from build123d import *

# Parameters (mm, degrees)
SKETCH1_R           = 6.25
BOSS_EXTRUDE1_DEPTH = 30
CUT_EXTRUDE3_DEPTH  = 15
SKETCH9_W           = 12.5
SKETCH9_H           = 25
BOSS_EXTRUDE2_DEPTH = 3
SKETCH11_W          = 10.933781676
SKETCH11_H          = 25
SKETCH11_W_2        = 11.938681189
CUT_EXTRUDE4_DEPTH  = 34
SKETCH12_R          = 6.25
BOSS_EXTRUDE3_DEPTH = 5
CHAMFER1_SIZE       = 1


with BuildPart() as part:
    # Sketch1 → Boss-Extrude1 (new body)
    with BuildSketch(Plane.XY):
        Circle(SKETCH1_R)
    extrude(amount=BOSS_EXTRUDE1_DEPTH)

    # Sketch8 → Cut-Extrude3 (cut)
    with BuildSketch(Plane(origin=(0, 0, 0), x_dir=(-1, 0, 0), z_dir=(0, 0, -1))):
        with BuildLine():
            Line((-1.616322988, 2.1), (1.616322988, 2.1))
            ThreePointArc((1.616322988, 2.1), (0, -2.65), (-1.616322988, 2.1))
        make_face()
    extrude(amount=-CUT_EXTRUDE3_DEPTH, mode=Mode.SUBTRACT)

    # Sketch9 → Boss-Extrude2 (add)
    with BuildSketch(Plane.XY.offset(30)):
        Rectangle(SKETCH9_W, SKETCH9_H)
    extrude(amount=BOSS_EXTRUDE2_DEPTH)

    # Sketch10 → Revolve1 (revolve)
    with BuildSketch(Plane(origin=(0, 0, 0), x_dir=(0, 0, -1), z_dir=(1, 0, 0))):
        Polygon((-30, 12.5), (-30, 0), (-17.5, 0), align=None)
    revolve(axis=Axis((0, 0, 63.541170981), (0, 0, 1)))

    # Sketch11 → Cut-Extrude4 (cut, through all)
    with BuildSketch(Plane.XY.offset(33)):
        with Locations((-11.716890838, 0)):
            Rectangle(SKETCH11_W, SKETCH11_H)
        with Locations((12.219340595, 0)):
            Rectangle(SKETCH11_W_2, SKETCH11_H)
    extrude(amount=-CUT_EXTRUDE4_DEPTH, mode=Mode.SUBTRACT)

    # Sketch12 → Boss-Extrude3 (add)
    with BuildSketch(Plane.XY.offset(33)):
        Circle(SKETCH12_R)
    extrude(amount=BOSS_EXTRUDE3_DEPTH)

    # Chamfer1
    chamfer1_edges = [part.edges().sort_by_distance(p)[0] for p in [
        (-6.25, 0, 38),
    ]]
    chamfer(chamfer1_edges, length=CHAMFER1_SIZE)


solid = part.part
Could you check a few things on this model? Use its own coordinates, in mm. A direction names the side the tool comes from. Coordinates: 2 decimals unless noted, no trailing zeros. Order: outer loops, then holes, each group sorted by start corner. A loop starts at its lowest first (then second) coordinate and runs counter-clockwise, first axis right, second up.
Q1. Thinking about a two-plate mould opening in Y: for faces 1 (the flat face through (5, 12, 30)), 2 (the flat face through (0, 2.1, 7)), 3 (the conical face through (0.2, 8.7, 26.2)), 4 (the cylindrical face through (-0.09, -2.65, 7.4)), which applies, released by +Y, released by -Y, zero draft, split by the parting line, or undercut?
Q2. Suppose I cut it at B-B on z = 26. Please give me the cut outline in (x, y), and give its area (3 significant figures).
Q3. Please list where these lines run through material, in increasing order: L1, parallel to Y at x = 0, z = 9.5; L2, parallel to X at y = 0, z = 4; L3, parallel to Y at x = -1, z = 11.
Q4. Will these pins go through, and if not, where does the flat tip stop? pin 1 (4 mm diameter, centred on x = -3.5, y = 9.5, fed in from -Z); pin 2 (2 mm diameter, centred on x = 2, z = 6, fed in from +Y); pin 3 (1.5 mm diameter, centred on y = -3.5, z = 11.5, fed in from +X).
Q5. Suppose I cut it at A-A on z = 34.5. Please give me the cut outline in (x, y), and give its area (3 significant figures).
Q6. Which directions (+Z, -Z, +X, -X, +Y, -Y) give clear straight access to the entire face, cutting with the end or side of a thin tool? Please do faces 5 (the cylindrical face through (5.96, 1.88, 11.71)), 6 (the flat face through (0, -9, 33)), 7 (the flat face through (-5, 12, 30)).
Answer:
1. face 1: zero draft
1. face 2: undercut
1. face 3: released by +Y
1. face 4: undercut
2. outline: (-6.25, -5.76) arc R8.5 ccw to (6.25, -5.76) - (6.25, 5.76) arc R8.5 ccw to (-6.25, 5.76) - close
2. area: 191 mm2
3. L1: y = -6.25 to -2.65, 2.1 to 6.25
3. L2: x = -6.25 to -2.65, 2.65 to 6.25
3. L3: y = -6.17 to -2.45, 2.1 to 6.17
4. pin 1: stops at z = 25.62
4. pin 2: stops at y = 6.17
4. pin 3: stops at x = 5.61
5. outline: circle Ø12.5 at (0, 0)
5. area: 123 mm2
6. face 5: -Z
6. face 6: +Z, -Y
6. face 7: -Z, -X, +Y
